The drawing under review shows one solid part. Ordinate dimensions are in mm from its lowest x, y, z. Coordinates: 2 decimals unless noted, no trailing zeros. Order: outer loops, then holes, each group sorted by start corner. A loop starts at its lowest first (then second) coordinate and runs counter-clockwise, first axis right, second up. Notation, with made-up numbers: (-38, 38) - (-31, 38) arc R36 cw to (-31, 75) - close; hole circle Ø4 at (-4.5, 69.25). An arc over 180 degrees is marked (long way). Write each question's results on one line, items separated by ' | '. Start each with the question number.
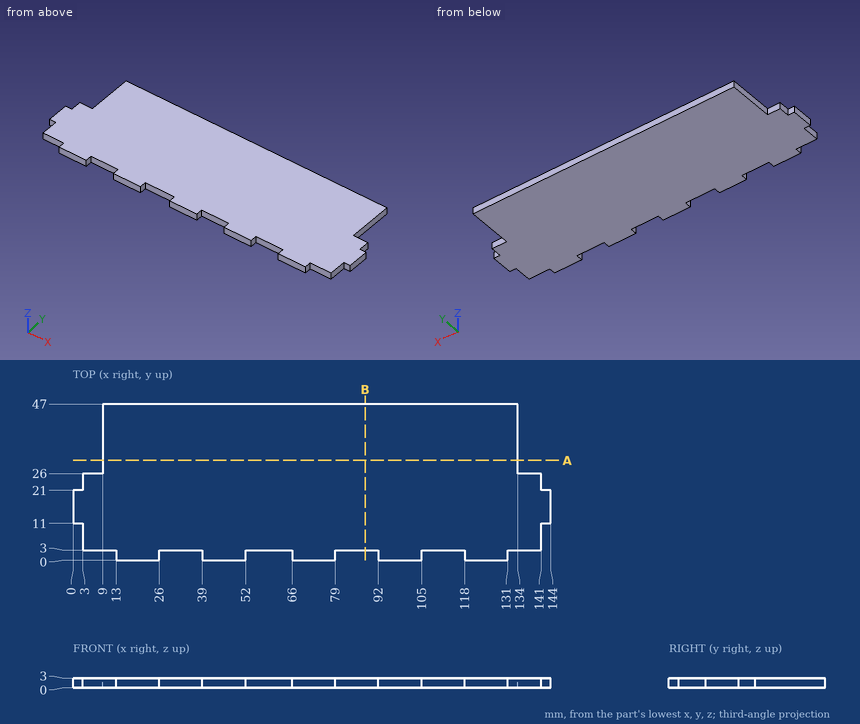
(1) Take a section at A-A (y = 30). State the section outline as (x, z) points.
(2) Take a section at B-B (x = 88). State the section outline as (y, z) points.
(3) To check wall thickness, follow line 1 along X through (y, z) = (39.5, 2.8); line 2 along X through (y, z) = (23, 2.6); line 3 along Y through (x, z) = (61.5, 2.7). State the ranges of each line that lie inside material, in increasing order. Write a range as [from, to].
(4) Clearance check with flat-ended pins moving along their axes: pin 1 (1.5 mm diameter, centred on x = 137, z = 2, fed in from +Y); pin 2 (0.9 mm diameter, centred on y = 1, z = 1, fed in from +X); pin 3 (0.9 mm diameter, centred on x = 60.5, z = 1.5, fed in from -Y). State where each tip first meets the part, or that it passes through.
Worked out:
1) outline: (9, 0) - (134, 0) - (134, 3) - (9, 3) - close
2) outline: (3, 0) - (47, 0) - (47, 3) - (3, 3) - close
3) line 1: [9, 134] | line 2: [3, 141] | line 3: [3, 47]
4) pin 1: y = 26 | pin 2: x = 131 | pin 3: y = 3
